from build123d import *

# Parameters (mm, degrees)
BOSS_EXTRUDE1_DEPTH = 4.5


with BuildPart() as part:
    # Sketch1 → Boss-Extrude1 (new body)
    with BuildSketch(Plane(origin=(0, 0, 0), x_dir=(1, 0, 0), z_dir=(0, 1, 0))):
        Polygon((11.714410298, 5), (11.714410298, -5), (10.785589702, -5), (10.785589702, -8.175), (-10.785589702, -8.175), (-10.785589702, -5), (-11.785589702, -5), (-11.785589702, 5), align=None)
        Polygon((10.785589702, 4), (10.785589702, -4), (9.785589702, -4), (9.785589702, -7.175), (-9.785589702, -7.175), (-9.785589702, -4), (-10.785589702, -4), (-10.785589702, 4), align=None, mode=Mode.SUBTRACT)
    extrude(amount=BOSS_EXTRUDE1_DEPTH)


solid = part.part
Source: CAD feature listing. Evaluate the final solid. Frame: model axes, mm. A direction names the side the tool comes from. Give positions to 0.01 mm unless a question says otherwise; leave off trailing zeros. Write each loop counter-clockwise with the first axis right and the second up, starting at its lowest first coordinate (ties: lowest second). Pieces come first, ordered by that corner, then holes. Notation, with made-up numbers: M -8,26 L 20,26 A17 ccw 20,50 Z; hole C -37.75,11.25 d6. An arc over 180 degrees is marked long. Return JSON: item names as keys, results as strings. Group by question number.
1) Cut plane A-A, the plane x = 7.5. Output: boundary loops of the cut face in (y, z) (3 decimals), then the cut area to 3 significant figures.
2) Ray query, L1, parallel to X at y = 0.45, z = -2.25; L2, parallel to Z at x = 10.25, y = 4.15 (3 decimals); L3, parallel to Z at x = 4, y = 0.8 (3 decimals). Return the intervals inside material, ascending.
3) Cut plane B-B, the plane z = 0. Output: boundary loops of the cut face in (x, y).
4) Cut plane C-C, the plane y = 1.2. Output: boundary loops of the cut face in (x, z) (3 decimals), then the cut area to 3 significant figures.
5) First-contact query: pin 1 Ø6 at (x, z) = (-4.5, 1.5) entering from -Y (3 decimals); pin 2 Ø0.5 at (x, y) = (-11.5, 1.5) entering from +Z; pin 3 Ø1.6 at (y, z) = (3, 6) entering from +X. Flat tips, straight axial feed; report the tip coordinate or a pass-through.
6) Set-up query: faces 5 (the face through (11.714, 2, 0)), 6 (the face through (-10.786, 2, 7)), 7 (the face through (10.786, 2, 7)), 8 (the face through (-11.786, 2, 0)), 9 (the face through (-9.786, 2, 6)). Return all of +Z, -Z, +X, -X, +Y, -Y with unobstructed straight access to the full face (end or side cutting, diameter ignored); none if empty.
7) Draft query along Z for faces 1 (the face through (9.786, 2, 6)), 2 (the face through (0, 2, 8.175)), 3 (the face through (-10, 2, 4)), 4 (the face through (0.9, 0, 7.4)). Return one class per face: released by +Z, released by -Z, zero draft, split by the parting line, or undercut.
Data:
{
 "1": {"outline": "M 0,-5 L 4.5,-5 L 4.5,-4 L 0,-4 Z; M 0,7.175 L 4.5,7.175 L 4.5,8.175 L 0,8.175 Z", "area": "9.00 mm²"},
 "2": {"L1": "x = -11.79 to -10.79, 10.79 to 11.71", "L2": "z = -5 to -4, 4 to 8.175", "L3": "z = -5 to -4, 7.175 to 8.175"},
 "3": {"outline": "M -11.79,0 L -10.79,0 L -10.79,4.5 L -11.79,4.5 Z; M 10.79,0 L 11.71,0 L 11.71,4.5 L 10.79,4.5 Z"},
 "4": {"outline": "M -11.786,-5 L 11.714,-5 L 11.714,5 L 10.786,5 L 10.786,8.175 L -10.786,8.175 L -10.786,5 L -11.786,5 Z; hole M -10.786,-4 L 10.786,-4 L 10.786,4 L 9.786,4 L 9.786,7.175 L -9.786,7.175 L -9.786,4 L -10.786,4 Z", "area": "68.8 mm²"},
 "5": {"pin 1": "passes through", "pin 2": "stops at z = 5", "pin 3": "stops at x = 10.79"},
 "6": {"face 5": "+Z, -Z, +X, +Y, -Y", "face 6": "+Z, -X, +Y, -Y", "face 7": "+Z, +X, +Y, -Y", "face 8": "+Z, -Z, -X, +Y, -Y", "face 9": "+Y, -Y"},
 "7": {"face 1": "undercut", "face 2": "released by +Z", "face 3": "undercut", "face 4": "zero draft"}
}
